Drawing for the job (mm, zero at the part's lowest x, y, z). Coordinates: 2 decimals unless noted, no trailing zeros. Loops run counter-clockwise (first coordinate to the right, second up) from the corner with the lowest first, then second, coordinate; pieces in that order, holes last. Notation, with made-up numbers: (48.5, 56) - (76.5, 56) arc R19 cw to (76.5, 67) - close; hole circle Ø11 at (-18, 2). An arc over 180 degrees is marked (long way). Put each result on its own line as item: value.
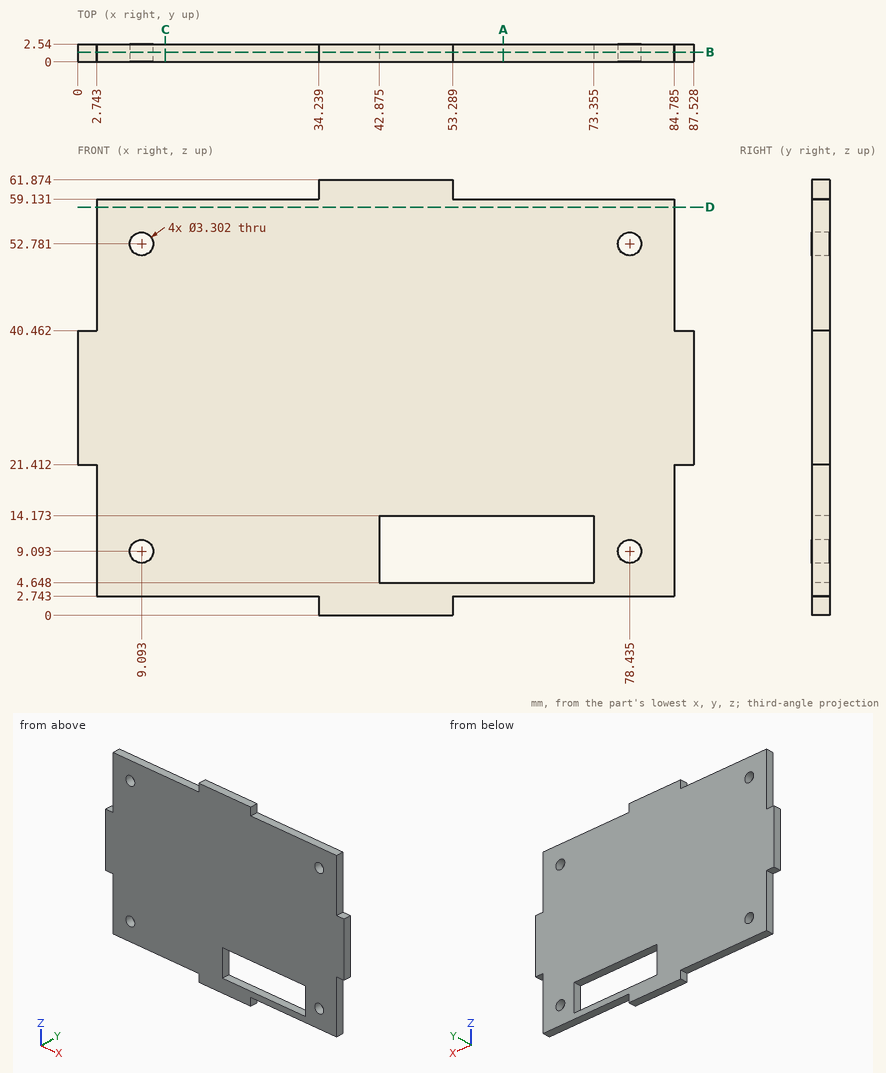
Q1. Slice it at B-B, the plane y = 1.4. Give the cut face in (x, z) (1 decimal).
Determined:
outline: (0, 21.4) - (2.7, 21.4) - (2.7, 2.7) - (34.2, 2.7) - (34.2, 0) - (53.3, 0) - (53.3, 2.7) - (84.8, 2.7) - (84.8, 21.4) - (87.5, 21.4) - (87.5, 40.5) - (84.8, 40.5) - (84.8, 59.1) - (53.3, 59.1) - (53.3, 61.9) - (34.2, 61.9) - (34.2, 59.1) - (2.7, 59.1) - (2.7, 40.5) - (0, 40.5) - close; hole circle Ø3.3 at (9.1, 9.1); hole circle Ø3.3 at (9.1, 52.8); hole (42.9, 4.6) - (73.4, 4.6) - (73.4, 14.2) - (42.9, 14.2) - close; hole circle Ø3.3 at (78.4, 9.1); hole circle Ø3.3 at (78.4, 52.8)
Q2. Pin check, flat tips, straight feed: pin 1 Ø2.5 at (x, z) = (9.09, 52.78) entering from +Y; pin 2 Ø0.8 at (x, y) = (1, 1) entering from +Z; pin 3 Ø1.3 at (y, z) = (2, 8) entering from +X (1 decimal); pin 4 Ø0.8 at (y, z) = (1.5, 1) entering from -X. Stop position of each tip, or through.
Determined:
pin 1: through
pin 2: z = 40.46
pin 3: x = 84.8
pin 4: x = 34.24
Q3. Slice it at D-D, the plane z = 58. Give the cut face in (x, y) (1 decimal).
Determined:
outline: (2.7, 0) - (84.8, 0) - (84.8, 2.5) - (2.7, 2.5) - close
Q4. Slice it at A-A, the plane x = 60.5. Give the cut face in (y, z).
Determined:
outline: (0, 2.74) - (2.54, 2.74) - (2.54, 4.65) - (0, 4.65) - close; (0, 14.17) - (2.54, 14.17) - (2.54, 59.13) - (0, 59.13) - close
Q5. Slice it at C-C, the plane x = 12.5. Give the cut face in (y, z).
Determined:
outline: (0, 2.74) - (2.54, 2.74) - (2.54, 59.13) - (0, 59.13) - close
Q6. Wall check: L1, parallel to Z at x = 44.5, y = 1.2 (1 decimal); L2, parallel to X at y = 2.2, z = 8.5 (1 decimal); L3, parallel to Z at x = 9, y = 1.85 (1 decimal). Give the ranges that are in metal, low to high. Write a range as from..to.
Determined:
L1: 0..4.6, 14.2..61.9
L2: 2.7..7.6, 10.6..42.9, 73.4..76.9, 80..84.8
L3: 2.7..7.4, 10.7..51.1, 54.4..59.1
